```python
from build123d import *

# Parameters (mm, degrees)
F0_W     = 28.5
F0_H     = 9
F0_R     = 1.525
F1_DEPTH = 7.5
F2_W     = 10.5
F2_H     = 9
F3_DEPTH = 3.5
F4_R     = 2.5
F5_SIZE2 = 1.5
F5_SIZE  = 1.5


with BuildPart() as f1:
    # F0 (on Top) → F1 (new body)
    with BuildSketch(Plane.XY):
        Rectangle(F0_W, F0_H)
        with Locations((-9.75, 0)):
            Circle(F0_R, mode=Mode.SUBTRACT)
        with Locations((9.75, 0)):
            Circle(F0_R, mode=Mode.SUBTRACT)
    extrude(amount=F1_DEPTH)

    # F2 (on face) → F3 (cut)
    with BuildSketch(Plane.XY.offset(7.5)):
        Rectangle(F2_W, F2_H)
    extrude(amount=-F3_DEPTH, mode=Mode.SUBTRACT)

    # F4
    f4_edges = [f1.edges().sort_by_distance(p)[0] for p in [
        (14.25, -4.5, 3.75),
        (14.25, 4.5, 3.75),
        (-14.25, -4.5, 3.75),
        (-14.25, 4.5, 3.75),
    ]]
    fillet(f4_edges, radius=F4_R)

    # F5
    f5_edges = [f1.edges().sort_by_distance(p)[0] for p in [
        (-11.275, 0, 0),
        (8.225, 0, 0),
    ]]
    chamfer(f5_edges, length=F5_SIZE, length2=F5_SIZE2)


solid = f1.part
```
Here's how the part is built. I have some questions about the finished solid (model axes, mm). A direction names the side the tool comes from. Give positions to 0.01 mm unless a question says otherwise; leave off trailing zeros. Loops run counter-clockwise (first coordinate to the right, second up) from the corner with the lowest first, then second, coordinate; pieces in that order, holes last. Notation, with made-up numbers: M 5,7.5 L 32,7.5 A22 cw 32,45.5 Z; hole C 20,-4.75 d11. An arc over 180 degrees is marked long. Use one line per item in the form item = value. Start each with the question number.
Q1. Will these pins go through, and if not, where does the flat tip stop? pin 1 Ø4.5 at (x, y) = (-0.5, 1) entering from +Z; pin 2 Ø4 at (x, y) = (9.75, 0) entering from -Z (3 decimals).
Q2. If we section it at B-B (y = 0): Write out the boundary of the cut face in (x, z) (3 decimals), then the cut area to 3 significant figures.
Q3. If we section it at C-C (x = -9.75): Write out the boundary of the cut face in (y, z) (3 decimals).
Q4. Thinking about a two-plate mould opening in Y: for faces 1 (the cylindrical face through (13.498, 3.787, 3.802)), 2 (the cylindrical face through (11.16, -0.58, 4.46)), 3 (the flat face through (5.25, 0, 6)), 4 (the cylindrical face through (-8.34, -0.58, 4.46)), which applies, +Y half, -Y half, draft (parallel to the pull), parting line (faces both ways), or undercut?
Q5. If we section it at D-D (z = 1.25): Write out the boundary of the cut face in (x, y) (3 decimals).
Q6. If we section it at A-A (z = 7): Write out the boundary of the cut face in (x, y) (3 decimals), then the cut area to 3 significant figures.
Q7. Which directions (+Z, -Z, +X, -X, +Y, -Y) give clear straight access to the entire face, cutting with the end or side of a thin tool? Please do faces 5 (the flat face through (8, 0, 7.5)), 6 (the flat face through (0, 0, 4)).
Q8. I need wall thicknesses on line 1 along Y through (x, z) = (-9.75, 5.35) (3 decimals); line 2 along X through (y, z) = (0.75, 6.25); line 3 along X through (y, z) = (-3, 7). Which ranges of each line are inside material? Lowest first, please.
Taken from the geometry:
q1.pin_1 = 4
q1.pin_2 = 1.025
q2.outline = M -14.25,0 L -12.775,0 L -11.275,1.5 L -11.275,7.5 L -14.25,7.5 Z; M -8.225,1.5 L -6.725,0 L 6.725,0 L 8.225,1.5 L 8.225,7.5 L 5.25,7.5 L 5.25,4 L -5.25,4 L -5.25,7.5 L -8.225,7.5 Z; M 11.275,1.5 L 12.775,0 L 14.25,0 L 14.25,7.5 L 11.275,7.5 Z
q2.area = 127 mm^2
q3.outline = M -4.5,0 L -3.025,0 L -1.525,1.5 L -1.525,7.5 L -4.5,7.5 Z; M 1.525,1.5 L 3.025,0 L 4.5,0 L 4.5,7.5 L 1.525,7.5 Z
q4.face_1 = +Y half
q4.face_2 = undercut
q4.face_3 = draft
q4.face_4 = undercut
q5.outline = M -14.25,-2 A2.5 ccw -11.75,-4.5 L 11.75,-4.5 A2.5 ccw 14.25,-2 L 14.25,2 A2.5 ccw 11.75,4.5 L -11.75,4.5 A2.5 ccw -14.25,2 Z; hole C -9.75,0 d3.55; hole C 9.75,0 d3.55
q6.outline = M -14.25,-2 A2.5 ccw -11.75,-4.5 L -5.25,-4.5 L -5.25,4.5 L -11.75,4.5 A2.5 ccw -14.25,2 Z; M 5.25,-4.5 L 11.75,-4.5 A2.5 ccw 14.25,-2 L 14.25,2 A2.5 ccw 11.75,4.5 L 5.25,4.5 Z; hole C -9.75,0 d3.05; hole C 9.75,0 d3.05
q6.area = 142 mm^2
q7.face_5 = +Z, +X, -X, +Y, -Y
q7.face_6 = +Z, +Y, -Y
q8.line_1 = -4.5 to -1.525, 1.525 to 4.5
q8.line_2 = -14.25 to -11.08, -8.42 to -5.25, 5.25 to 8.42, 11.08 to 14.25
q8.line_3 = -14.04 to -5.25, 5.25 to 14.04
